Input: part model. Units: mm. Frame: model coordinates. A direction names the side the tool comes from. Round coordinates to 2 decimals unless told otherwise and drop trailing zeros. Write each loop counter-clockwise with the first axis right and the second up, starting at its lowest first coordinate (ties: lowest second). Pieces come first, ordered by that corner, then holes. Notation, with made-up numbers: (-31, -21) -> (27, -21) arc R17 ccw to (27, 4) -> close; hole circle Ø6 at (-25.5, 61). An arc over 180 degrees is marked (long way). Use CSV: the item, a comma, the result in double quotes.
Autodesk Inventor part; units mm, degrees
ref_plane "YZ Plane" through (0, 0, 0) normal (1, 0, 0) x (0, 1, 0)
ref_plane "XZ Plane" through (0, 0, 0) normal (0, 1, 0) x (-1, 0, 0)
ref_plane "XY Plane" through (0, 0, 0) normal (0, 0, 1) x (1, 0, 0)
sketch "Sketch1" plane through (0, 0, 0) normal (0, 0, 1) x (1, 0, 0)
  arc A0 (2.25, 0) -> (-2.25, 0) centre (0, 0) ccw
  line L0 (0, 0) -> (-2.25, 0) construction
  line L1 (0, 0) -> (2.25, 0) construction
  line L2 (5.5, 0) -> (-5.5, 0)
  line L3 (-5.5, 0) -> (-5.5, 5.5)
  line L4 (-5.5, 5.5) -> (5.5, 5.5)
  line L5 (5.5, 5.5) -> (5.5, 0)
  line L6 (-19, 0) -> (75.5, 0)
  circle A1 centre (57, 30) radius 2.25
  circle A2 centre (57, 30) radius 5
  line L7 (-5.5, 5.5) -> (52, 35)
  line L8 (52, 35) -> (57, 35)
  line L9 (57, 25) -> (50, 25)
  line L10 (50, 25) -> (50, 0)
  line L11 (-5.5, 0) -> (50, 0)
  point P0 (52, 30)
  point P1 (-2.25, 0)
  point P2 (50, 0)
  dimension "d0" = 2.25
  dimension "d1" = 180
  dimension "d2" = 11
  dimension "d3" = 5.5
  dimension "d4" = 4.5
  dimension "d5" = 10
  dimension "d6" = 25
  dimension "d7" = 90
  dimension "d8" = 55.5
  dimension "d42" = 64.6258
  dimension "d43" = 5
extrude "Extrusion1" add sketch "Sketch1" along normal blind 10 contours A0 L2 L3 L4 L5 | L5 L4 L7 L8 A2 L9 L10 L6 | A2
mirror "Mirror1" about plane through (0, 0, 0) normal (0, 1, 0)
fillet "Fillet1" radius 2 2 edges at (50, 25, 5) (50, -25, 5)
sketch "Sketch2" plane through (0, 0, 10) normal (0, 0, 1) x (1, 0, 0)
  circle A0 centre (0, 0) radius 2.25
  line L0 (0, 0) -> (69.506, 0)
  line L1 (0, 0) -> (0, 32.0889)
  line L2 (41.5, 21) -> (8.5, 4) construction
  line L3 (40.4696, 23.0002) -> (7.4696, 6.0002)
  line L4 (9.5304, 1.9998) -> (42.5304, 18.9998)
  arc A1 (42.5304, 18.9998) -> (40.4696, 23.0002) centre (41.5, 21) ccw
  arc A2 (7.4696, 6.0002) -> (9.5304, 1.9998) centre (8.5, 4) ccw
  line L5 (41.5, 21) -> (8.5, 4) construction
  line L6 (39.8972, 24.1114) -> (6.8972, 7.1114)
  line L7 (10.1028, 0.8886) -> (43.1028, 17.8886)
  arc A3 (43.1028, 17.8886) -> (39.8972, 24.1114) centre (41.5, 21) ccw
  arc A4 (6.8972, 7.1114) -> (10.1028, 0.8886) centre (8.5, 4) ccw
  arc A5 (52, 25) -> (50, 23) centre (52, 23) ccw construction
  line L8 (52, 25) -> (57, 25) construction
  arc A6 (57, 25) -> (57, 35) centre (57, 30) ccw construction
  line L9 (57, 35) -> (52, 35) construction
  line L10 (52, 35) -> (-5.5, 5.5) construction
  line L11 (-5.5, 5.5) -> (-5.5, -5.5) construction
  line L12 (52, -35) -> (-5.5, -5.5) construction
  line L13 (57, -35) -> (52, -35) construction
  arc A7 (57, -35) -> (57, -25) centre (57, -30) ccw construction
  line L14 (52, -25) -> (57, -25) construction
  arc A8 (50, -23) -> (52, -25) centre (52, -23) ccw construction
  line L15 (50, 23) -> (50, -23) construction
  circle A9 centre (57, -30) radius 2.25 construction
  circle A10 centre (0, 0) radius 2.25 construction
  circle A11 centre (57, 30) radius 2.25 construction
  point P0 (25, 12.5)
  point P1 (25, 12.5)
  dimension "d15" = 4.5
  dimension "d16" = 7
  dimension "d38" = 47
  dimension "d39" = 14
  dimension "d40" = 4
  dimension "d41" = 21
extrude "Extrusion2" cut sketch "Sketch2" against normal blind 3 contours A3 L7 A4 L6
sketch "Sketch3" plane through (0, 0, 10) normal (0, 0, 1) x (1, 0, 0)
  arc A0 (42.5304, 18.9998) -> (40.4696, 23.0002) centre (41.5, 21) ccw
  arc A1 (7.4696, 6.0002) -> (9.5304, 1.9998) centre (8.5, 4) ccw
  line L0 (41.5, 21) -> (8.5, 4) construction
  line L1 (40.4696, 23.0002) -> (7.4696, 6.0002)
  line L2 (9.5304, 1.9998) -> (42.5304, 18.9998)
  arc A2 (42.5304, 18.9998) -> (40.4696, 23.0002) centre (41.5, 21) ccw
  arc A3 (7.4696, 6.0002) -> (9.5304, 1.9998) centre (8.5, 4) ccw
  point P0 (0, 0)
  point P1 (25, 12.5)
  dimension "d19" = 4.5
extrude "Extrusion3" cut sketch "Sketch3" against normal blind 10
mirror "Mirror2" about plane through (0, 0, 0) normal (0, 1, 0) of "Extrusion2", "Extrusion1", "Extrusion3"
sketch "Sketch4" plane through (0, 0, 10) normal (0, 0, 1) x (1, 0, 0)
  circle A0 centre (40, 5) radius 1.75
  point P0 (0, 0)
  dimension "d24" = 3.5
hole "Hole1" at (40, 5, 10) direction (0, 0, -1) diameter 2.459 end through all
mirror "Mirror6" about plane through (0, 0, 0) normal (0, 1, 0) of "Hole1", "Extrusion2", "Extrusion3"
chamfer "Chamfer1" distance 2 angle 45 1 edges at (52, 35, 5)
chamfer "Chamfer2" distance 2 angle 45 1 edges at (52, -35, 5)
properties part number "V structure"
Item 1: Section query B-B on x = 8.5. Return the cut outline in (y, z), plus the area to 3 significant figures.
Worked answers:
outline,"(-12.68, 0) -> (-6.53, 0) -> (-6.53, 7) -> (-7.94, 7) -> (-7.94, 10) -> (-12.68, 10) -> close; (-1.75, 0) -> (1.75, 0) -> (1.75, 7) -> (0.5, 7) -> (0.5, 10) -> (-0.5, 10) -> (-0.5, 7) -> (-1.75, 7) -> close; (6.53, 0) -> (12.68, 0) -> (12.68, 10) -> (7.94, 10) -> (7.94, 7) -> (6.53, 7) -> close"
area,"142 mm²"
Item 2: Line query: line 1 (X direction, y = -5, z = 5); line 2 (Y direction, x = 58, z = 4); line 3 (Y direction, x = 20, z = 6). Output: solid intervals per line, ascending.
Worked answers:
line 1,"x = -5.5 to 6.48, 15.35 to 38.77, 41.23 to 50"
line 2,"y = -34.9 to -32.02, -27.98 to -25.1, 25.1 to 27.98, 32.02 to 34.9"
line 3,"y = -18.58 to -12.46, -7.39 to 7.39, 12.46 to 18.58"
Item 3: Set-up query: faces 4 (the face through (25.8, 10.38, 3.55)), 5 (the face through (31, 0, 0)), 6 (the face through (55, 25, 5)), 7 (the face through (27, -10, 7)). Return all of +Z, -Z, +X, -X, +Y, -Y with unobstructed straight access to the full face (end or side cutting, diameter ignored); none if empty.
Worked answers:
face 4,"+Z, -Z"
face 5,"-Z, +X, -X, +Y, -Y"
face 6,"+Z, -Z, +X"
face 7,"+Z"
Item 4: Section query C-C on y = -9. Return the cut outline in (x, z), plus the area to 3 significant figures.
Worked answers:
outline,"(1.32, 0) -> (13.29, 0) -> (13.29, 7) -> (10.56, 7) -> (10.56, 10) -> (1.32, 10) -> close; (23.12, 0) -> (50, 0) -> (50, 10) -> (25.85, 10) -> (25.85, 7) -> (23.12, 7) -> close"
area,"372 mm²"
Item 5: Pull-direction query (Y, two-part tool) for faces 1 (the face through (22.75, -19.994, 4.93)), 2 (the face through (31, 0, 10)), 3 (the face through (54.752, -30.099, 4.93)); classes: +Y half, -Y half, draft (parallel to the pull), parting line (faces both ways), or undercut.
Worked answers:
face 1,"-Y half"
face 2,"draft"
face 3,"undercut"
Item 6: Section query D-D on x = 53. Return the cut outline in (y, z).
Worked answers:
outline,"(-34.76, 0) -> (-25, 0) -> (-25, 10) -> (-34.76, 10) -> close; (25, 0) -> (34.76, 0) -> (34.76, 10) -> (25, 10) -> close"
Item 7: Section query A-A on z = 3.5. Return the cut outline in (x, y), plus the area to 3 significant figures.
Worked answers:
outline,"(-5.5, -5.5) -> (50.22, -34.09) -> (54, -35) -> (57, -35) arc R5 ccw to (57, -25) -> (52, -25) arc R2 cw to (50, -23) -> (50, 23) arc R2 cw to (52, 25) -> (57, 25) arc R5 ccw to (57, 35) -> (54, 35) -> (50.22, 34.09) -> (-5.5, 5.5) -> close; hole circle Ø4.5 at (0, 0); hole (7.47, -6) -> (40.47, -23) arc R2.25 ccw to (42.53, -19) -> (9.53, -2) arc R2.25 ccw to start; hole (7.47, 6) arc R2.25 ccw to (9.53, 2) -> (42.53, 19) arc R2.25 ccw to (40.47, 23) -> close; hole circle Ø2.46 at (40, -5); hole circle Ø2.46 at (40, 5); hole circle Ø4.5 at (57, -30); hole circle Ø4.5 at (57, 30)"
area,"1,980 mm²"
Item 8: First-contact query: pin 1 Ø1.5 at (x, z) = (37.5, 5) entering from -Y; pin 2 Ø4 at (x, z) = (42, 3) entering from -Y; pin 3 Ø12 at (x, y) = (40, -3) entering from -Z; pin 4 Ø4 at (x, y) = (57, 30) entering from -Z. Flat tips, straight axial feed; report the tip coordinate or a pass-through.
Worked answers:
pin 1,"stops at y = -27.95"
pin 2,"stops at y = -30.9"
pin 3,"stops at z = 0"
pin 4,"passes through"
